from build123d import *

# Parameters (mm, degrees)
ESBO_O1_R                = 4
RESSALTO_EXTRUS_O1_DEPTH = 10
RESSALTO_EXTRUS_O2_DEPTH = 2
ESBO_O2_R                = 1.6
CORTE_EXTRUS_O1_DEPTH    = 10


with BuildPart() as part:
    # Esboço1 → Ressalto-extrusão1 (new body)
    with BuildSketch(Plane.XY):
        with BuildLine():
            Line((6, 4.5), (6, 55.5))
            ThreePointArc((6, 55.5), (-3.354101966, 66.708203932), (0, 52.5))
            Line((0, 52.5), (0, 7.5))
            ThreePointArc((0, 7.5), (-3.354101966, -6.708203932), (6, 4.5))
        make_face()
        Circle(ESBO_O1_R, mode=Mode.SUBTRACT)
        with Locations((0, 60)):
            Circle(ESBO_O1_R, mode=Mode.SUBTRACT)
    extrude(amount=RESSALTO_EXTRUS_O1_DEPTH)

    # Esboço3 → Ressalto-extrusão2 (add)
    with BuildSketch(Plane.XY.offset(10)):
        with BuildLine():
            Line((0, 52.5), (0, 7.5))
            ThreePointArc((0, 7.5), (-3.354101966, -6.708203932), (6, 4.5))
            Line((6, 4.5), (6, 55.5))
            ThreePointArc((6, 55.5), (-3.354101966, 66.708203932), (0, 52.5))
        make_face()
    extrude(amount=RESSALTO_EXTRUS_O2_DEPTH)

    # Esboço2 → Corte-extrusão1 (cut)
    with BuildSketch(Plane.ZY):
        with Locations(Location((6, 30, 0), (0, 0, 270))):
            Circle(ESBO_O2_R)
    extrude(amount=-CORTE_EXTRUS_O1_DEPTH, mode=Mode.SUBTRACT)


solid = part.part
Source: CAD feature listing. Evaluate the final solid. Frame: model axes, mm. A direction names the side the tool comes from. Round coordinates to 2 decimals unless told otherwise and drop trailing zeros. Loops run counter-clockwise (first coordinate to the right, second up) from the corner with the lowest first, then second, coordinate; pieces in that order, holes last. Notation, with made-up numbers: M 26,56.25 L 38,56.25 A23 cw 38,81.25 Z; hole C 29,10 d6. An arc over 180 degrees is marked long. Return JSON: item names as keys, results as strings. Group by question number.
1. Section query A-A on z = 6. Output: boundary loops of the cut face in (x, y).
2. Mould query, pull axis Y, two halves, no side actions, for faces 4 (the face through (0, 30, 3)), 5 (the face through (-0.867, 56.095, 4.93)), 6 (the face through (2, 31, 0)). Classes: released by +Y, released by -Y, zero draft, split by the parting line, or undercut.
3. Section query D-D on x = -1.75. Output: boundary loops of the cut face in (y, z), and give its area (3 significant figures).
4. Material intervals for line 1 along Y through (x, z) = (0.25, 8); line 2 along Z through (x, y) = (3.5, 30); line 3 along Y through (x, z) = (-0.5, 9.5), sorted ascending. Write a range as from..to.
5. Pin query (flat end, axial travel): pin 1 (3.5 mm diameter, centred on y = 22, z = 8.5, fed in from +X); pin 2 (4 mm diameter, centred on y = 35.5, z = 5, fed in from -X); pin 3 (3 mm diameter, centred on x = -4.5, z = 8, fed in from -Y). Return the tip coordinate at first contact, or that it passes through.
6. Section query B-B on y = 30. Output: boundary loops of the cut face in (x, z), and give its area (3 significant figures).
7. Section query C-C on z = 2.75. Output: boundary loops of the cut face in (x, y), and give its area (3 significant figures).
8. Reachability of faces 1 (the face through (6, 30, 3)), 2 (the face through (2, 31, 12)), 3 (the face through (0, 0, 10)) from +Z, -Z, +X, -X, +Y, -Y: full face, straight path, thin tool, end or side. Return the list, or none.
Checks:
{
 "1": {"outline": "M 0,7.5 A7.5 ccw long 6,4.5 L 6,28.4 L 0,28.4 Z; M 0,31.6 L 6,31.6 L 6,55.5 A7.5 ccw long 0,52.5 Z; hole C 0,0 d8; hole C 0,60 d8"},
 "2": {"face 4": "undercut", "face 5": "undercut", "face 6": "zero draft"},
 "3": {"outline": "M -7.29,0 L -3.6,0 L -3.6,10 L 3.6,10 L 3.6,0 L 7.29,0 L 7.29,12 L -7.29,12 Z; M 52.71,0 L 56.4,0 L 56.4,10 L 63.6,10 L 63.6,0 L 67.29,0 L 67.29,12 L 52.71,12 Z", "area": "206 mm²"},
 "4": {"line 1": "y = -7.5..-3.99, 3.99..56.01, 63.99..67.5", "line 2": "z = 0..4.4, 7.6..12", "line 3": "y = -7.48..-3.97, 3.97..7.48, 52.52..56.03, 63.97..67.48"},
 "5": {"pin 1": "stops at x = 6", "pin 2": "stops at x = 0", "pin 3": "stops at y = -6.87"},
 "6": {"outline": "M 0,0 L 6,0 L 6,4.4 L 0,4.4 Z; M 0,7.6 L 6,7.6 L 6,12 L 0,12 Z", "area": "52.8 mm²"},
 "7": {"outline": "M 0,7.5 A7.5 ccw long 6,4.5 L 6,55.5 A7.5 ccw long 0,52.5 Z; hole C 0,0 d8; hole C 0,60 d8", "area": "534 mm²"},
 "8": {"face 1": "+Z, -Z, +X", "face 2": "+Z, +X, -X, +Y, -Y", "face 3": "-Z"}
}
